Can you work these out from the model? Positions are in its coordinate system, mm. A direction names the side the tool comes from. Give positions to 0.01 mm unless a question says otherwise; leave off trailing zeros. Write each loop counter-clockwise with the first axis right and the second up, starting at its lowest first coordinate (ties: lowest second). Pieces come first, ordered by that corner, then holes. Notation, with made-up numbers: (-6.75, -5.5) -> (51.25, -5.5) arc R7 cw to (51.25, -0.5) -> close; hole circle Ø8 at (81, 79). An arc over 180 degrees is marked (long way). Answer as CSV lines item,"result". Start each with the question number.
1. I'm going to push flat-ended pins straight in: P1, Ø7, axis at x = -10, z = 33, coming from the +Y side; P2, Ø6, axis at y = 10, z = 13, coming from the -X side; P3, Ø4.5, axis at x = -10, y = 10, coming from the -Z side; P4, Ø1.5, axis at y = -5, z = 57.5, coming from the +X side. Where does each tip first touch, or does it pass through?
2. If we section it at C-C on y = -7: Write out the boundary of the cut face in (x, z) (3 decimals).
3. On a 3-axis mill with a long thin cutter (end or side, diameter ignored), from which of +Z, -Z, +X, -X, +Y, -Y can I reach the whole of each face in a straight line? I mean faces 1 (the face through (4, 3, 60)), 2 (the face through (5.07, 8.37, 15.12)), 3 (the face through (-2, -4, 60)). Say none if no direction works.
4. If we mould it in two halves opening along Z, with no side actions, what happens to faces 4 (the face through (1, 3, 100)), 5 (the face through (10, 8, 51)), 6 (the face through (-6.96, -9.71, 56.97))? For each: pulls with the +Z half, pulls with the -Z half, needs draft (parallel to the pull), parting line crosses it, or undercut.
5. I need wall thicknesses on line 1 (Y direction, x = 0.5, z = 17.5); line 2 (Z direction, x = -10, y = -3.2) (3 decimals); line 3 (Y direction, x = 2.7, z = 90). Which ranges of each line are inside material? Lowest first, please. Write a range as [from, to].
6. If we section it at B-B on x = 2: Write out the boundary of the cut face in (y, z) (3 decimals), plus the area to 3 significant figures.
7. If we section it at D-D on z = 83: Write out the boundary of the cut face in (x, y), plus the area to 3 significant figures.
8. If we section it at A-A on z = 73: Write out the boundary of the cut face in (x, y) (3 decimals), plus the area to 3 significant figures.
```python
from build123d import *

# Parameters (mm, degrees)
SKETCH1_R                      = 2.7
BOSS_EXTRUDE1_DEPTH            = 3
BOSS_EXTRUDE2_DEPTH            = 100
CUT_EXTRUDE1_DEPTH             = 20
CUT_EXTRUDE2_DEPTH             = 20
SKETCH4_R                      = 9
BOSS_EXTRUDE3_DEPTH            = 6
BOSS_EXTRUDE3_TAPER            = 35
CUT_EXTRUDE3_REACH             = 26
SKETCH4_3_R                    = 2.675
SKETCH4_3_R_2                  = 2.7
CUT_EXTRUDE3_DIRECTION_2_REACH = 8
SKETCH5_R                      = 2.675
SKETCH5_R_2                    = 2.7
CUT_EXTRUDE4_DEPTH             = 10


with BuildPart() as part:
    # Sketch1 → Boss-Extrude1 (new body)
    with BuildSketch(Plane.XY):
        with BuildLine():
            Line((-1.267766953, 0), (-20, 0))
            Line((-20, 0), (-20, 20))
            Line((-20, 20), (0, 20))
            Line((0, 20), (0, 1.267766953))
            ThreePointArc((0, 1.267766953), (0.038060234, 1.076425237), (0.146446609, 0.914213562))
            Line((0.146446609, 0.914213562), (0.530330086, 0.530330086))
            ThreePointArc((0.530330086, 0.530330086), (0.530330086, -0.530330086), (-0.530330086, -0.530330086))
            Line((-0.530330086, -0.530330086), (-0.914213562, -0.146446609))
            ThreePointArc((-0.914213562, -0.146446609), (-1.076425237, -0.038060234), (-1.267766953, 0))
        make_face()
        with Locations((-10, 10)):
            Circle(SKETCH1_R, mode=Mode.SUBTRACT)
    extrude(amount=BOSS_EXTRUDE1_DEPTH)

    # Sketch1<4> → Boss-Extrude2 (add)
    with BuildSketch(Plane.XY):
        with BuildLine():
            ThreePointArc((-1.267766953, 0), (-1.076425237, -0.038060234), (-0.914213562, -0.146446609))
            Line((-0.914213562, -0.146446609), (-0.530330086, -0.530330086))
            ThreePointArc((-0.530330086, -0.530330086), (0.530330086, -0.530330086), (0.530330086, 0.530330086))
            Line((0.530330086, 0.530330086), (0.146446609, 0.914213562))
            ThreePointArc((0.146446609, 0.914213562), (0.038060234, 1.076425237), (0, 1.267766953))
            Line((0, 1.267766953), (0, 20))
            Line((0, 20), (4, 20))
            Line((4, 20), (4, -4))
            Line((4, -4), (-20, -4))
            Line((-20, -4), (-20, 0))
            Line((-20, 0), (-1.267766953, 0))
        make_face()
    extrude(amount=BOSS_EXTRUDE2_DEPTH)

    # Sketch2 → Cut-Extrude1 (cut)
    with BuildSketch(Plane(origin=(0, 20, 0), x_dir=(1, 0, 0), z_dir=(0, 1, 0))):
        Polygon((0, -3), (0.5, -3), (0, -4), align=None)
    extrude(amount=-CUT_EXTRUDE1_DEPTH, mode=Mode.SUBTRACT)

    # Sketch3 → Cut-Extrude2 (cut)
    with BuildSketch(Plane.ZY.offset(20)):
        Polygon((3, 0), (3, -0.5), (4, 0), align=None)
    extrude(amount=-CUT_EXTRUDE2_DEPTH, mode=Mode.SUBTRACT)

    # Sketch4 → Boss-Extrude3 (add)
    with BuildSketch(Plane(origin=(4, 0, 0), x_dir=(0, 0, -1), z_dir=(1, 0, 0))):
        with Locations((-13, 10)):
            Circle(SKETCH4_R)
        with Locations((-33, 10)):
            Circle(SKETCH4_R)
        with Locations((-53, 10)):
            Circle(SKETCH4_R)
        with Locations((-73, 10)):
            Circle(SKETCH4_R)
    boss_extrude3 = extrude(amount=BOSS_EXTRUDE3_DEPTH, taper=BOSS_EXTRUDE3_TAPER)

    # Cut-Extrude3: up to this face of the body (flat: up to its plane)
    cut_extrude3_end = Plane(part.part.faces().sort_by_distance((0, 10.633883476, 52))[0])
    # Sketch4<3> → Cut-Extrude3 (cut, up to the picked face)
    with BuildSketch(Plane(origin=(4, 0, 0), x_dir=(0, 0, -1), z_dir=(1, 0, 0)), mode=Mode.PRIVATE) as cut_extrude3_sk1:
        with Locations((-13, 10)):
            Circle(SKETCH4_3_R)
    cut_extrude3_tool1 = split(extrude(cut_extrude3_sk1.sketch, amount=-CUT_EXTRUDE3_REACH, mode=Mode.PRIVATE), bisect_by=cut_extrude3_end, keep=Keep.BOTH, mode=Mode.PRIVATE)
    add(cut_extrude3_tool1.solids().sort_by_distance((4, 10, 13))[0], mode=Mode.SUBTRACT)
    # Sketch4<3> → Cut-Extrude3 (cut, up to the picked face)
    with BuildSketch(Plane(origin=(4, 0, 0), x_dir=(0, 0, -1), z_dir=(1, 0, 0)), mode=Mode.PRIVATE) as cut_extrude3_sk2:
        with Locations((-33, 10)):
            Circle(SKETCH4_3_R)
    cut_extrude3_tool2 = split(extrude(cut_extrude3_sk2.sketch, amount=-CUT_EXTRUDE3_REACH, mode=Mode.PRIVATE), bisect_by=cut_extrude3_end, keep=Keep.BOTH, mode=Mode.PRIVATE)
    add(cut_extrude3_tool2.solids().sort_by_distance((4, 10, 33))[0], mode=Mode.SUBTRACT)
    # Sketch4<3> → Cut-Extrude3 (cut, up to the picked face)
    with BuildSketch(Plane(origin=(4, 0, 0), x_dir=(0, 0, -1), z_dir=(1, 0, 0)), mode=Mode.PRIVATE) as cut_extrude3_sk3:
        with Locations((-53, 10)):
            Circle(SKETCH4_3_R)
    cut_extrude3_tool3 = split(extrude(cut_extrude3_sk3.sketch, amount=-CUT_EXTRUDE3_REACH, mode=Mode.PRIVATE), bisect_by=cut_extrude3_end, keep=Keep.BOTH, mode=Mode.PRIVATE)
    add(cut_extrude3_tool3.solids().sort_by_distance((4, 10, 53))[0], mode=Mode.SUBTRACT)
    # Sketch4<3> → Cut-Extrude3 (cut, up to the picked face)
    with BuildSketch(Plane(origin=(4, 0, 0), x_dir=(0, 0, -1), z_dir=(1, 0, 0)), mode=Mode.PRIVATE) as cut_extrude3_sk4:
        with Locations((-73, 10)):
            Circle(SKETCH4_3_R)
    cut_extrude3_tool4 = split(extrude(cut_extrude3_sk4.sketch, amount=-CUT_EXTRUDE3_REACH, mode=Mode.PRIVATE), bisect_by=cut_extrude3_end, keep=Keep.BOTH, mode=Mode.PRIVATE)
    add(cut_extrude3_tool4.solids().sort_by_distance((4, 10, 73))[0], mode=Mode.SUBTRACT)
    # Sketch4<3> → Cut-Extrude3 (cut, up to the picked face)
    with BuildSketch(Plane(origin=(4, 0, 0), x_dir=(0, 0, -1), z_dir=(1, 0, 0)), mode=Mode.PRIVATE) as cut_extrude3_sk5:
        with Locations((-90, 10)):
            Circle(SKETCH4_3_R_2)
    cut_extrude3_tool5 = split(extrude(cut_extrude3_sk5.sketch, amount=-CUT_EXTRUDE3_REACH, mode=Mode.PRIVATE), bisect_by=cut_extrude3_end, keep=Keep.BOTH, mode=Mode.PRIVATE)
    add(cut_extrude3_tool5.solids().sort_by_distance((4, 10, 90))[0], mode=Mode.SUBTRACT)

    # Cut-Extrude3 direction 2: up to this face of the body (flat: up to its plane)
    cut_extrude3_direction_2_end = Plane(part.part.faces().sort_by_distance((10, 10, 73))[0])
    # Sketch4<3> → Cut-Extrude3 direction 2 (cut, up to the picked face)
    with BuildSketch(Plane(origin=(4, 0, 0), x_dir=(0, 0, -1), z_dir=(1, 0, 0)), mode=Mode.PRIVATE) as cut_extrude3_direction_2_sk1:
        with Locations((-13, 10)):
            Circle(SKETCH4_3_R)
    cut_extrude3_direction_2_tool1 = split(extrude(cut_extrude3_direction_2_sk1.sketch, amount=CUT_EXTRUDE3_DIRECTION_2_REACH, mode=Mode.PRIVATE), bisect_by=cut_extrude3_direction_2_end, keep=Keep.BOTH, mode=Mode.PRIVATE)
    add(cut_extrude3_direction_2_tool1.solids().sort_by_distance((4, 10, 13))[0], mode=Mode.SUBTRACT)
    # Sketch4<3> → Cut-Extrude3 direction 2 (cut, up to the picked face)
    with BuildSketch(Plane(origin=(4, 0, 0), x_dir=(0, 0, -1), z_dir=(1, 0, 0)), mode=Mode.PRIVATE) as cut_extrude3_direction_2_sk2:
        with Locations((-33, 10)):
            Circle(SKETCH4_3_R)
    cut_extrude3_direction_2_tool2 = split(extrude(cut_extrude3_direction_2_sk2.sketch, amount=CUT_EXTRUDE3_DIRECTION_2_REACH, mode=Mode.PRIVATE), bisect_by=cut_extrude3_direction_2_end, keep=Keep.BOTH, mode=Mode.PRIVATE)
    add(cut_extrude3_direction_2_tool2.solids().sort_by_distance((4, 10, 33))[0], mode=Mode.SUBTRACT)
    # Sketch4<3> → Cut-Extrude3 direction 2 (cut, up to the picked face)
    with BuildSketch(Plane(origin=(4, 0, 0), x_dir=(0, 0, -1), z_dir=(1, 0, 0)), mode=Mode.PRIVATE) as cut_extrude3_direction_2_sk3:
        with Locations((-53, 10)):
            Circle(SKETCH4_3_R)
    cut_extrude3_direction_2_tool3 = split(extrude(cut_extrude3_direction_2_sk3.sketch, amount=CUT_EXTRUDE3_DIRECTION_2_REACH, mode=Mode.PRIVATE), bisect_by=cut_extrude3_direction_2_end, keep=Keep.BOTH, mode=Mode.PRIVATE)
    add(cut_extrude3_direction_2_tool3.solids().sort_by_distance((4, 10, 53))[0], mode=Mode.SUBTRACT)
    # Sketch4<3> → Cut-Extrude3 direction 2 (cut, up to the picked face)
    with BuildSketch(Plane(origin=(4, 0, 0), x_dir=(0, 0, -1), z_dir=(1, 0, 0)), mode=Mode.PRIVATE) as cut_extrude3_direction_2_sk4:
        with Locations((-73, 10)):
            Circle(SKETCH4_3_R)
    cut_extrude3_direction_2_tool4 = split(extrude(cut_extrude3_direction_2_sk4.sketch, amount=CUT_EXTRUDE3_DIRECTION_2_REACH, mode=Mode.PRIVATE), bisect_by=cut_extrude3_direction_2_end, keep=Keep.BOTH, mode=Mode.PRIVATE)
    add(cut_extrude3_direction_2_tool4.solids().sort_by_distance((4, 10, 73))[0], mode=Mode.SUBTRACT)
    # Sketch4<3> → Cut-Extrude3 direction 2 (cut, up to the picked face)
    with BuildSketch(Plane(origin=(4, 0, 0), x_dir=(0, 0, -1), z_dir=(1, 0, 0)), mode=Mode.PRIVATE) as cut_extrude3_direction_2_sk5:
        with Locations((-90, 10)):
            Circle(SKETCH4_3_R_2)
    cut_extrude3_direction_2_tool5 = split(extrude(cut_extrude3_direction_2_sk5.sketch, amount=CUT_EXTRUDE3_DIRECTION_2_REACH, mode=Mode.PRIVATE), bisect_by=cut_extrude3_direction_2_end, keep=Keep.BOTH, mode=Mode.PRIVATE)
    add(cut_extrude3_direction_2_tool5.solids().sort_by_distance((4, 10, 90))[0], mode=Mode.SUBTRACT)

    # Mirror1: Boss-Extrude3 across plane
    add(boss_extrude3.mirror(Plane(origin=(0, 0, 0), x_dir=(0, 0, 1), z_dir=(0.707106781, 0.707106781, 0))))

    # Sketch5 → Cut-Extrude4 (cut)
    with BuildSketch(Plane.XZ.offset(10)):
        with Locations((-10, 13)):
            Circle(SKETCH5_R)
        with Locations((-10, 90)):
            Circle(SKETCH5_R_2)
        with Locations((-10, 33)):
            Circle(SKETCH5_R)
        with Locations((-10, 53)):
            Circle(SKETCH5_R)
        with Locations((-10, 73)):
            Circle(SKETCH5_R)
    extrude(amount=-CUT_EXTRUDE4_DEPTH, mode=Mode.SUBTRACT)


solid = part.part
```
Computed values:
1,P1,"stops at y = 0"
1,P2,"stops at x = 0"
1,P3,"passes through"
1,P4,"stops at x = -2.28"
2,outline,"circle Ø13.799 at (-10, 13); circle Ø13.799 at (-10, 33); circle Ø13.799 at (-10, 53); circle Ø13.799 at (-10, 73); hole circle Ø5.35 at (-10, 13); hole circle Ø5.35 at (-10, 33); hole circle Ø5.35 at (-10, 53); hole circle Ø5.35 at (-10, 73)"
3,face 1,"+X"
3,face 2,"+X, -X"
3,face 3,"-Y"
4,face 4,"pulls with the +Z half"
4,face 5,"needs draft"
4,face 6,"undercut"
5,line 1,"y = [-4, -0.56], [0.56, 20]"
5,line 2,"z = [0, 10.325], [15.675, 30.325], [35.675, 50.325], [55.675, 70.325], [75.675, 87.3], [92.7, 100]"
5,line 3,"y = [-4, 7.3], [12.7, 20]"
6,outline,"(-4, 0) -> (20, 0) -> (20, 100) -> (-4, 100) -> close; hole circle Ø5.4 at (10, 90); hole circle Ø5.35 at (10, 13); hole circle Ø5.35 at (10, 33); hole circle Ø5.35 at (10, 53); hole circle Ø5.35 at (10, 73)"
6,area,"2,290 mm2"
7,outline,"(-20, -4) -> (4, -4) -> (4, 20) -> (0, 20) -> (0, 1.27) arc R0.5 ccw to (0.15, 0.91) -> (0.53, 0.53) arc R0.75 cw to (-0.53, -0.53) -> (-0.91, -0.15) arc R0.5 ccw to (-1.27, 0) -> (-20, 0) -> close"
7,area,"175 mm2"
8,outline,"(-20, -4) -> (-19, -4) -> (-14.799, -10) -> (-12.675, -10) -> (-12.675, 0) -> (-20, 0) -> close; (-7.325, -10) -> (-5.201, -10) -> (-1, -4) -> (4, -4) -> (4, 1) -> (10, 5.201) -> (10, 7.325) -> (0, 7.325) -> (0, 1.268) arc R0.5 ccw to (0.146, 0.914) -> (0.53, 0.53) arc R0.75 cw to (-0.53, -0.53) -> (-0.914, -0.146) arc R0.5 ccw to (-1.268, 0) -> (-7.325, 0) -> close; (0, 12.675) -> (10, 12.675) -> (10, 14.799) -> (4, 19) -> (4, 20) -> (0, 20) -> close"
8,area,"233 mm2"
